CAD build for the part. Positions are in the model's coordinates, mm. Face numbers are marked on the shaded views. Round coordinates to 2 decimals unless told otherwise and drop trailing zeros. Order: outer loops, then holes, each group sorted by start corner. A loop starts at its lowest first (then second) coordinate and runs counter-clockwise, first axis right, second up. Notation, with made-up numbers: (64.25, 89.5) -> (80.25, 89.5) arc R17 cw to (80.25, 114.5) -> close; hole circle Ø6 at (-27.5, 0). An arc over 180 degrees is marked (long way). Return JSON: item names as keys, results as strings. Group by question number.
Q1. Cut at A-A (y = 35). Write the cut outline in (x, z).
Q2. Mould opens along Z. For the marked faces 1, 2 and 3 say: +Z half, -Z half, draft (parallel to the pull), parting line (faces both ways), or undercut.
Q3. Probe line 1 along Z through (x, y) = (0, 34); line 2 along Z through (x, y) = (-0.25, -18.5); line 3 along X through (y, z) = (-24, 3). List the from-to ranges inside material, lowest first.
Q4. Flat gauge pins, fed straight in: pin 1 (2 mm diameter, centred on x = 3, y = 17, fed in from +Z); pin 2 (4 mm diameter, centred on x = 0, z = 0, fed in from +Y). Where does each tip first touch, or does it go through?
Q5. Cut at B-B (y = 15). Write the cut outline in (x, z).
Autodesk Inventor part; units mm, degrees
ref_plane "YZ Plane" through (0, 0, 0) normal (1, 0, 0) x (0, 1, 0)
ref_plane "XZ Plane" through (0, 0, 0) normal (0, 1, 0) x (-1, 0, 0)
ref_plane "XY Plane" through (0, 0, 0) normal (0, 0, 1) x (1, 0, 0)
sketch "Sketch1" plane through (0, 0, 0) normal (0, 1, 0) x (-1, 0, 0)
  circle A0 centre (0, 0) radius 5
  dimension "d0" = 10
extrude "Extrusion1" add sketch "Sketch1" along normal mid plane 80
chamfer "Chamfer1" distance 1 angle 45 1 edges at (5, -40, 0)
hole "Hole3" at (0, 40, 0) direction (0, -1, 0) diameter 4.917 depth 17.1 tip angle 118
properties part number "suporte-barra" material "Aluminium AW-7020"
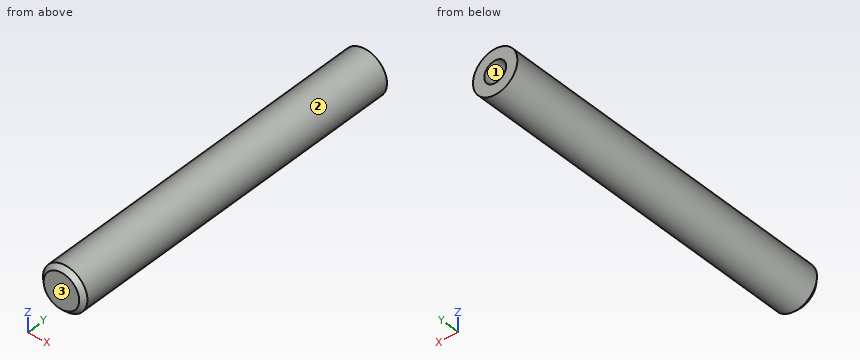
Solution:
{
 "1": {"outline": "circle Ø10 at (0, 0); hole circle Ø4.92 at (0, 0)"},
 "2": {"face 1": "undercut", "face 2": "parting line", "face 3": "draft"},
 "3": {"line 1": "z = -5 to -2.46, 2.46 to 5", "line 2": "z = -4.99 to 4.99", "line 3": "x = -4 to 4"},
 "4": {"pin 1": "stops at z = 4.58", "pin 2": "stops at y = 22.62"},
 "5": {"outline": "circle Ø10 at (0, 0)"}
}
